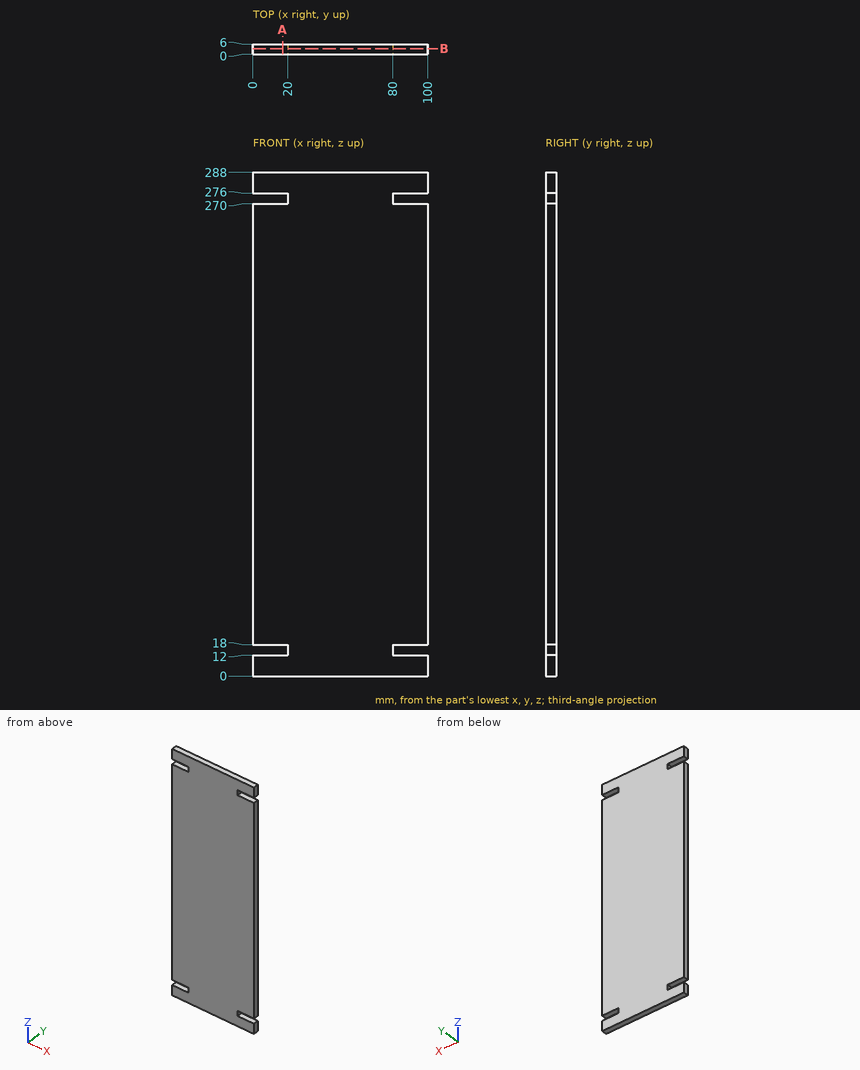
Here's the drawing with two shaded views (mm, measured from the low corner). I have some questions. Round coordinates to 2 decimals unless told otherwise and drop trailing zeros. Loops run counter-clockwise (first coordinate to the right, second up) from the corner with the lowest first, then second, coordinate; pieces in that order, holes last.
Item 1: Please list where this line runs through material, in increasing order: L1, parallel to Z at x = 12, y = 1.45.
Item 2: Suppose I cut it at B-B, the plane y = 3.35. Write out the boundary of the cut face in (x, z), then the cut area to 3 significant figures.
Item 3: Will this pin go through, and if not, where does the flat tip stop? pin 1 Ø1.8 at (y, z) = (1.5, 273.5) entering from -X.
Item 4: Suppose I cut it at A-A, the plane x = 17. Write out the boundary of the cut face in (y, z).
Reported:
1. L1: z = 0 to 12, 18 to 270, 276 to 288
2. outline: (0, 0) - (100, 0) - (100, 12) - (80, 12) - (80, 18) - (100, 18) - (100, 270) - (80, 270) - (80, 276) - (100, 276) - (100, 288) - (0, 288) - (0, 276) - (20, 276) - (20, 270) - (0, 270) - (0, 18) - (20, 18) - (20, 12) - (0, 12) - close
2. area: 28,300 mm2
3. pin 1: stops at x = 20
4. outline: (0, 0) - (6, 0) - (6, 12) - (0, 12) - close; (0, 18) - (6, 18) - (6, 270) - (0, 270) - close; (0, 276) - (6, 276) - (6, 288) - (0, 288) - close
